from build123d import *

# Parameters (mm, degrees)
F0_W     = 1212.85
F0_H     = 273.05
F1_DEPTH = 19.05
F2_W     = 19.05
F2_H     = 273.05
F2_H_2   = 254
F3_DEPTH = 9.525
F4_W     = 1174.75
F4_H     = 6.35
F5_DEPTH = 9.525


with BuildPart() as f1:
    # F0 (on Top) → F1 (new body)
    with BuildSketch(Plane.XY):
        with Locations((606.425, 136.525)):
            Rectangle(F0_W, F0_H)
    extrude(amount=F1_DEPTH)

    # F2 (on face) → F3 (cut)
    with BuildSketch(Plane(origin=(0, 0, 0), x_dir=(1, 0, 0), z_dir=(0, 0, -1))):
        with Locations((9.525, -136.525)):
            Rectangle(F2_W, F2_H)
        with Locations((307.975, -146.05)):
            Rectangle(F2_W, F2_H_2)
        with Locations((606.425, -146.05)):
            Rectangle(F2_W, F2_H_2)
        with Locations((904.875, -146.05)):
            Rectangle(F2_W, F2_H_2)
        with Locations((1203.325, -136.525)):
            Rectangle(F2_W, F2_H)
    extrude(amount=-F3_DEPTH, mode=Mode.SUBTRACT)

    # F4 (on face) → F5 (cut)
    with BuildSketch(Plane(origin=(0, 0, 0), x_dir=(1, 0, 0), z_dir=(0, 0, -1))):
        with Locations((606.425, -269.875)):
            Rectangle(F4_W, F4_H)
    extrude(amount=-F5_DEPTH, mode=Mode.SUBTRACT)


solid = f1.part
The model under review builds one solid part; all positions refer to its coordinate system, in mm. Give positions to 0.01 mm unless a question says otherwise; leave off trailing zeros. Loops run counter-clockwise (first coordinate to the right, second up) from the corner with the lowest first, then second, coordinate; pieces in that order, holes last. Notation, with made-up numbers: (41.25, 10) -> (100.25, 10) arc R9 cw to (100.25, 16) -> close; hole circle Ø6 at (-39, 40.25). An arc over 180 degrees is marked (long way). Answer as a JSON object with one key per item and string values. Group by question number.
Q1. Insertion check: pin 1 (5 mm diameter, centred on x = 311.5, z = 4.5, fed in from +Y); pin 2 (3 mm diameter, centred on x = 1030.5, y = 171.5, fed in from -Z); pin 3 (10.5 mm diameter, centred on y = 101.5, z = 3.5, fed in from -X); pin 4 (7.5 mm diameter, centred on x = 197.5, z = 5, fed in from +Y). Each pin has a flat end and moves straight along its axis. Give the tip position at first contact, or say it passes through.
Q2. Wall thickness on line 1 along X through (y, z) = (84.5, 1.5); line 2 along Y through (x, z) = (195.5, 2); line 3 along Y through (x, z) = (303, 2.75): over which ranges is each line inside the solid? List them lowest first.
Q3. Take a section at A-A (y = 218). Write out the cut boundary in (x, z) (3 decimals), plus the area to 3 significant figures.
Q4. Draft analysis for pull direction X (two halves, no side actions). For faces 1 (the flat face through (598, 138, 19.05)), 2 (the flat face through (604, 207, 9.525)), state which applies: pulls with the +X half, pulls with the -X half, needs draft (parallel to the pull), parting line crosses it, or undercut.
Answer below:
{
 "1": {"pin 1": "stops at y = 19.05", "pin 2": "stops at z = 0", "pin 3": "stops at x = 19.05", "pin 4": "stops at y = 266.7"},
 "2": {"line 1": "x = 19.05 to 298.45, 317.5 to 596.9, 615.95 to 895.35, 914.4 to 1193.8", "line 2": "y = 0 to 266.7", "line 3": "y = 0 to 19.05"},
 "3": {"outline": "(0, 9.525) -> (19.05, 9.525) -> (19.05, 0) -> (298.45, 0) -> (298.45, 9.525) -> (317.5, 9.525) -> (317.5, 0) -> (596.9, 0) -> (596.9, 9.525) -> (615.95, 9.525) -> (615.95, 0) -> (895.35, 0) -> (895.35, 9.525) -> (914.4, 9.525) -> (914.4, 0) -> (1193.8, 0) -> (1193.8, 9.525) -> (1212.85, 9.525) -> (1212.85, 19.05) -> (0, 19.05) -> close", "area": "22,200 mm2"},
 "4": {"face 1": "needs draft", "face 2": "undercut"}
}
